Can you work these out from the model? Positions are in its coordinate system, mm. A direction names the side the tool comes from. Coordinates: 2 decimals unless noted, no trailing zeros. Order: outer loops, then holes, each group sorted by start corner. A loop starts at its lowest first (then second) coordinate and runs counter-clockwise, first axis right, second up. Notation, with made-up numbers: (-34, 72.25) - (-25, 72.25) arc R12 cw to (-25, 77.25) - close; hole circle Ø6 at (-9.5, -24.75). An arc over 180 degrees is marked (long way). Return JSON: item names as keys, results as strings. Group by question number.
1) Imagine slicing it at A-A (z = -514). Write out the boundary of the cut face in (x, y) (3 decimals), and give its area (3 significant figures).
2) Imagine slicing it at B-B (y = 3.25). Write out the boundary of the cut face in (x, z).
3) If I drill on line 1 along Z through (x, y) = (12.7, -2.15) (3 decimals); line 2 along X through (y, z) = (-2.25, -88.9) (3 decimals); line 3 along Z through (x, y) = (12.7, -1.1) (3 decimals), over which ranges is the centre line in solid material (lowest first)?
4) Which directions (+Z, -Z, +X, -X, +Y, -Y) give clear straight access to the entire face, cutting with the end or side of a thin tool? Please do faces 1 (the face through (13, -3.175, -273)), 2 (the face through (13, 0, -281)).
5) For pin 1 Ø2 at (x, y) = (15.5, 7) entering from -Z; pin 2 Ø12 at (x, z) = (5.5, -259) entering from +Y; pin 3 Ø3 at (x, y) = (13.5, 5.5) entering from +Z, each with a flat end and sliding along its axis, tell me the tip position at first contact or that it passes through.
```python
from build123d import *

# Parameters (mm, degrees)
BOSS_EXTRUDE1_DEPTH = 25.4
SKETCH2_R           = 3.175
CUT_EXTRUDE1_DEPTH  = 4.175
FILLET1_R           = 2.54


with BuildPart() as part:
    # Sketch1 → Boss-Extrude1 (new body)
    with BuildSketch(Plane(origin=(0, 0, 0), x_dir=(0, 0, -1), z_dir=(1, 0, 0))):
        with BuildLine():
            Line((0, 0), (-21.997045256, 12.7))
            Line((-21.997045256, 12.7), (-23.584545256, 9.950369343))
            Line((-23.584545256, 9.950369343), (-1.5875, -2.749630657))
            ThreePointArc((-1.5875, -2.749630657), (-0.821750468, -3.066814498), (0, -3.175))
            Line((0, -3.175), (553.1612, -3.175))
            Line((553.1612, -3.175), (553.1612, 0))
            Line((553.1612, 0), (0, 0))
        make_face()
    extrude(amount=BOSS_EXTRUDE1_DEPTH)

    # Sketch2 → Cut-Extrude1 (cut, through all)
    with BuildSketch(Plane(origin=(0, 0, 0), x_dir=(1, 0, 0), z_dir=(0, 1, 0))):
        with Locations((12.7, 88.9)):
            Circle(SKETCH2_R)
        with Locations((12.7, 464.2612)):
            Circle(SKETCH2_R)
    extrude(amount=-CUT_EXTRUDE1_DEPTH, mode=Mode.SUBTRACT)

    # Fillet1
    fillet1_edges = [part.edges().sort_by_distance(p)[0] for p in [
        (25.4, 11.325184671, 22.790795256),
        (12.7, 0, 0),
        (25.4, -1.5875, -553.1612),
        (0, -1.5875, -553.1612),
        (0, 11.325184671, 22.790795256),
    ]]
    fillet(fillet1_edges, radius=FILLET1_R)


solid = part.part
```
Calculated:
{
 "1": {"outline": "(0, -3.175) - (25.4, -3.175) - (25.4, 0) - (0, 0) - close", "area": "80.6 mm2"},
 "2": {"outline": "(0, 5.63) - (25.4, 5.63) - (25.4, 11.98) - (0, 11.98) - close"},
 "3": {"line 1": "-553.161 to -467.436, -461.086 to -92.075, -85.725 to 2.626", "line 2": "0 to 9.525, 15.875 to 25.4", "line 3": "-553.161 to -467.436, -461.086 to -92.075, -85.725 to 4.445"},
 "4": {"face 1": "+Z, -Z, +X, -X, -Y", "face 2": "-Z, +X, -X, +Y"},
 "5": {"pin 1": "z = 10.39", "pin 2": "y = 0", "pin 3": "z = 18.47"}
}
